```python
from build123d import *

# Parameters (mm, degrees)
F0_W     = 25.4
F0_H     = 50.8
F1_DEPTH = 25.4
F2_R     = 5.08
F3_R     = 3.31416
F4_DEPTH = 71.882
F5_W     = 6.293828
F5_H     = 0.982571
F5_W_2   = 5.419478
F5_H_2   = 3.787311
F5_W_3   = 14.692617
F5_H_3   = 7.307336
F6_DEPTH = 25.4
F7_R     = 3.064351
F8_DEPTH = 14.986


with BuildPart() as f1:
    # F0 (on Top) → F1 (new body)
    with BuildSketch(Plane.XY):
        with Locations((-12.7, 25.4)):
            Rectangle(F0_W, F0_H)
    extrude(amount=F1_DEPTH)

    # F2
    f2_edges = [f1.edges().sort_by_distance(p)[0] for p in [
        (0, 0, 12.7),
        (-25.4, 0, 12.7),
        (0, 50.8, 12.7),
        (-25.4, 50.8, 12.7),
    ]]
    fillet(f2_edges, radius=F2_R)

    # F3 (on face) → F4 (join)
    with BuildSketch(Plane.XY.offset(25.4)):
        with Locations((-12.072328, 15.729843)):
            Circle(F3_R)
    extrude(amount=F4_DEPTH)

    # F5 (on face) → F6 (join)
    with BuildSketch(Plane(origin=(-25.4, 0, 0), x_dir=(0, -1, 0), z_dir=(-1, 0, 0))):
        with Locations((-12.68953, 12.160792)):
            Rectangle(F5_W, F5_H)
        with Locations((-18.546183, 4.663679)):
            Rectangle(F5_W_2, F5_H_2)
        with Locations((-29.99346, 13.014776)):
            Rectangle(F5_W_3, F5_H_3)
    extrude(amount=F6_DEPTH)

    # F7 (on face) → F8 (join)
    with BuildSketch(Plane.XY.offset(16.668444)):
        with Locations((-40.764336, 31.40362)):
            Circle(F7_R)
    extrude(amount=F8_DEPTH)


solid = f1.part
```
Check sheet for the modelled part. Datum: model origin and axes. Units: mm. A direction names the side the tool comes from. Coordinates: 2 decimals unless noted, no trailing zeros. Loops run counter-clockwise (first coordinate to the right, second up) from the corner with the lowest first, then second, coordinate; pieces in that order, holes last.
1) Gauge pin test, flat ends, axial feed: pin 1 (4 mm diameter, centred on y = 11, z = 23, fed in from -X); pin 2 (5 mm diameter, centred on x = -40.5, y = 30.5, fed in from +Z); pin 3 (12 mm diameter, centred on y = 21.5, z = 60.5, fed in from -X). Record the tip position at first contact, or that the pin passes through.
2) Release check for a two-part mould opening along X. For faces 4 (the face through (-38, 28, 16.668)), 5 (the face through (-1.528, 1.449, 12.878)), 6 (the face through (-38, 13, 11.67)) record: released by +X, released by -X, zero draft, split by the parting line, or undercut.
3) Sectioned sample at C-C (y = 30). Record the boundary of the cut face in (x, z).
4) Access from +Z, -Z, +X, -X, +Y, -Y to the whole of each face (thin tool, end or side, straight path). Record for faces 1 (the face through (-38, 30, 9.361)), 2 (the face through (-38, 37.34, 13)), 3 (the face through (-41.429, 28.412, 24.057)).
5) Material ranges on probe 1 along Z at (x, y) = (-19, 12); probe 2 along X at (y, z) = (15.5, 59); probe 3 along Z at (x, y) = (-41, 26), recorded low to high.
6) Sectioned sample at A-A (x = -32). Record the boundary of the cut face in (y, z).
7) Sectioned sample at D-D (x = -39). Record the boundary of the cut face in (y, z).
8) Sectioned sample at B-B (x = -10.5). Record the boundary of the cut face in (y, z), and give its area (3 significant figures).
Check sheet entries:
1. pin 1: stops at x = -25.4
1. pin 2: stops at z = 31.65
1. pin 3: stops at x = -15.39
2. face 4: undercut
2. face 5: released by +X
2. face 6: zero draft
3. outline: (-50.8, 9.36) - (-25.4, 9.36) - (-25.4, 0) - (0, 0) - (0, 25.4) - (-25.4, 25.4) - (-25.4, 16.67) - (-38.04, 16.67) - (-38.04, 31.65) - (-43.49, 31.65) - (-43.49, 16.67) - (-50.8, 16.67) - close
4. face 1: -Z, -X, +Y, -Y
4. face 2: +Z, -Z, -X, +Y
4. face 3: +Z
5. probe 1: z = 0 to 25.4
5. probe 2: x = -15.38 to -8.77
5. probe 3: z = 9.36 to 16.67
6. outline: (9.54, 11.67) - (15.84, 11.67) - (15.84, 12.65) - (9.54, 12.65) - close; (15.84, 2.77) - (21.26, 2.77) - (21.26, 6.56) - (15.84, 6.56) - close; (22.65, 9.36) - (37.34, 9.36) - (37.34, 16.67) - (22.65, 16.67) - close
7. outline: (9.54, 11.67) - (15.84, 11.67) - (15.84, 12.65) - (9.54, 12.65) - close; (15.84, 2.77) - (21.26, 2.77) - (21.26, 6.56) - (15.84, 6.56) - close; (22.65, 9.36) - (37.34, 9.36) - (37.34, 16.67) - (33.91, 16.67) - (33.91, 31.65) - (28.9, 31.65) - (28.9, 16.67) - (22.65, 16.67) - close
8. outline: (0, 0) - (50.8, 0) - (50.8, 25.4) - (18.65, 25.4) - (18.65, 97.28) - (12.81, 97.28) - (12.81, 25.4) - (0, 25.4) - close
8. area: 1,710 mm2
